Autodesk Inventor part; units mm, degrees
ref_plane "YZ Plane" through (0, 0, 0) normal (1, 0, 0) x (0, 1, 0)
ref_plane "XZ Plane" through (0, 0, 0) normal (0, 1, 0) x (-1, 0, 0)
ref_plane "XY Plane" through (0, 0, 0) normal (0, 0, 1) x (1, 0, 0)
sketch "Sketch1" plane through (0, 0, 0) normal (0, 1, 0) x (-1, 0, 0)
  line L0 (-15, 0) -> (15, 0)
  line L1 (15, 0) -> (15, -66)
  line L2 (15, -66) -> (-15, -66)
  line L3 (-15, -66) -> (-15, 0)
  circle A0 centre (0, -8) radius 1.65
  circle A1 centre (0, -26) radius 1.65
  point P0 (0, 0)
  point P1 (0, 0)
  dimension "d0" = 66
  dimension "d1" = 30
  dimension "d2" = 3.3
  dimension "d3" = 3.3
  dimension "d4" = 18
  dimension "d5" = 8
extrude "Extrusion1" add sketch "Sketch1" along normal blind 10
chamfer "Chamfer1" distance 5 angle 45 2 edges at (15, 5, 0) (-15, 5, 0)
sketch "Sketch2" plane through (15, 0, -66) normal (0, 0, -1) x (-1, 0, 0)
  line L0 (0, 0) -> (30, 0)
  line L1 (30, 0) -> (30, 10)
  line L2 (0, 10) -> (30, 10)
  line L3 (0, 0) -> (0, 10)
  line L4 (15, 0) -> (15, -14)
  line L5 (15, -14) -> (61, -14)
  line L6 (61, -14) -> (15, 36.0799)
  line L7 (15, 0) -> (15, 57.2033) construction
  circle A0 centre (15, 36.0799) radius 11
  line L8 (-0.5, 20.5799) -> (30.5, 20.5799) construction
  line L9 (30.5, 20.5799) -> (30.5, 51.5799) construction
  line L10 (30.5, 51.5799) -> (-0.5, 51.5799) construction
  line L11 (-0.5, 51.5799) -> (-0.5, 20.5799) construction
  line L12 (-0.5, 20.5799) -> (30.5, 51.5799) construction
  line L13 (30.5, 20.5799) -> (-0.5, 51.5799) construction
  circle A1 centre (-0.5, 51.5799) radius 1.65
  circle A2 centre (30.5, 51.5799) radius 1.65
  circle A3 centre (30.5, 20.5799) radius 1.65
  circle A4 centre (-0.5, 20.5799) radius 1.65
  line L14 (-5.5, 0) -> (35.5, 0)
  line L15 (35.5, 0) -> (35.5, 60)
  line L16 (35.5, 60) -> (-5.5, 60)
  line L17 (-5.5, 60) -> (-5.5, 0)
  dimension "d11" = 14
  dimension "d12" = 46
  dimension "d13" = 68
  dimension "d14" = 22
  dimension "d15" = 31
  dimension "d16" = 31
  dimension "d17" = 3.3
  dimension "d18" = 60
  dimension "d19" = 41
extrude "Extrusion2" add sketch "Sketch2" against normal blind 8 contours L14 L17 L16 L15 L1 L2 L3
chamfer "Chamfer2" distance 5 angle 45 7 edges at (20.5, 60, -62) (-20.5, 60, -62) (20.5, 0, -62) (15, 5, -58) (-15, 5, -58) (-20.5, 0, -62) (0, 10, -58)
properties part number "SOPORTE_NEMA_2" material "Steel, Mild, Welded"
Read the model definition and answer for the solid it produces. Units are mm, in the model's axes. A direction names the side the tool comes from. Round coordinates to 2 decimals unless told otherwise and drop trailing zeros. Loops run counter-clockwise (first coordinate to the right, second up) from the corner with the lowest first, then second, coordinate; pieces in that order, holes last. Notation, with made-up numbers: (51, 83) - (91, 83) arc R17 cw to (91, 93) - close; hole circle Ø6 at (21.5, 27). An arc over 180 degrees is marked (long way). One line per question, with ' | ' between items. Start each with the question number.
Q1. Section C-C on y = 38.5 is taken. Give the vertices of the cut face in (x, z), plus the area to 3 significant figures.
Q2. Find the intervals of material crossed by L1, parallel to Y at x = -15.5, z = -60.5; L2, parallel to Y at x = 15, z = -62; L3, parallel to Z at x = -15.5, y = 34.5, in increasing order.
Q3. For faces 4 (the flat face through (15, 5, -29)), 5 (the flat face through (-15, 5, -29)), 6 (the flat face through (0, 24, -66)), determine the directions among +Z, -Z, +X, -X, +Y, -Y from which every point of the face is accessible in a straight line to the end or side of a thin tool.
Q4. For a pull along X with two mould halves and no side action, classify faces 1 (the flat face through (0, 5, 0)), 2 (the flat face through (13, 5, -3)), 3 (the cylindrical face through (14.61, 52.97, -62.06)) as +X half, -X half, draft (parallel to the pull), parting line (faces both ways), or undercut.
Q5. Section A-A on x = 0 is taken. Give the vertices of the cut face in (y, z), plus the area to 4 significant figures.
Q6. Flat-ended cylindrical pins translate along their axes: pin 1 (6 mm diameter, centred on x = 9, y = 24.5, fed in from +Z); pin 2 (11 mm diameter, centred on y = 3, z = -18.5, fed in from -X); pin 3 (3 mm diameter, centred on y = 5.5, z = -29, fed in from +X). Find the tip coordinate at first contact, or state that the pin passes through.
Q7. Section B-B on z = -26 is taken. Give the vertices of the cut face in (x, y), plus the area to 3 significant figures.
Q8. Section D-D on y = 6.5 is taken. Give the vertices of the cut face in (x, z), plus the area to 3 significant figures.
Established:
1) outline: (-20.5, -66) - (-10.73, -66) - (-10.73, -58) - (-20.5, -58) - close; (10.73, -66) - (20.5, -66) - (20.5, -58) - (10.73, -58) - close | area: 156 mm²
2) L1: 0 to 18.93, 22.23 to 49.93, 53.23 to 60 | L2: 0 to 19.01, 22.15 to 50.01, 53.15 to 60 | L3: -66 to -58
3) face 4: +Z, +X, +Y, -Y | face 5: +Z, -X, +Y, -Y | face 6: -Z, +X, -X, +Y, -Y
4) face 1: draft | face 2: +X half | face 3: undercut
5) outline: (0, -66) - (25.08, -66) - (25.08, -58) - (15, -58) - (10, -53) - (10, -27.65) - (0, -27.65) - close; (0, -24.35) - (10, -24.35) - (10, -9.65) - (0, -9.65) - close; (0, -6.35) - (10, -6.35) - (10, 0) - (0, 0) - close; (47.08, -66) - (60, -66) - (60, -58) - (47.08, -58) - close | area: 830.5 mm²
6) pin 1: z = -58 | pin 2: x = -15 | pin 3: x = 15
7) outline: (-15, 0) - (-1.65, 0) - (-1.65, 10) - (-15, 10) - close; (1.65, 0) - (15, 0) - (15, 10) - (1.65, 10) - close | area: 267 mm²
8) outline: (-20.5, -66) - (20.5, -66) - (20.5, -58) - (20, -58) - (15, -53) - (15, -5) - (10, 0) - (-10, 0) - (-15, -5) - (-15, -53) - (-20, -58) - (-20.5, -58) - close; hole circle Ø3.3 at (0, -26); hole circle Ø3.3 at (0, -8) | area: 2,050 mm²
